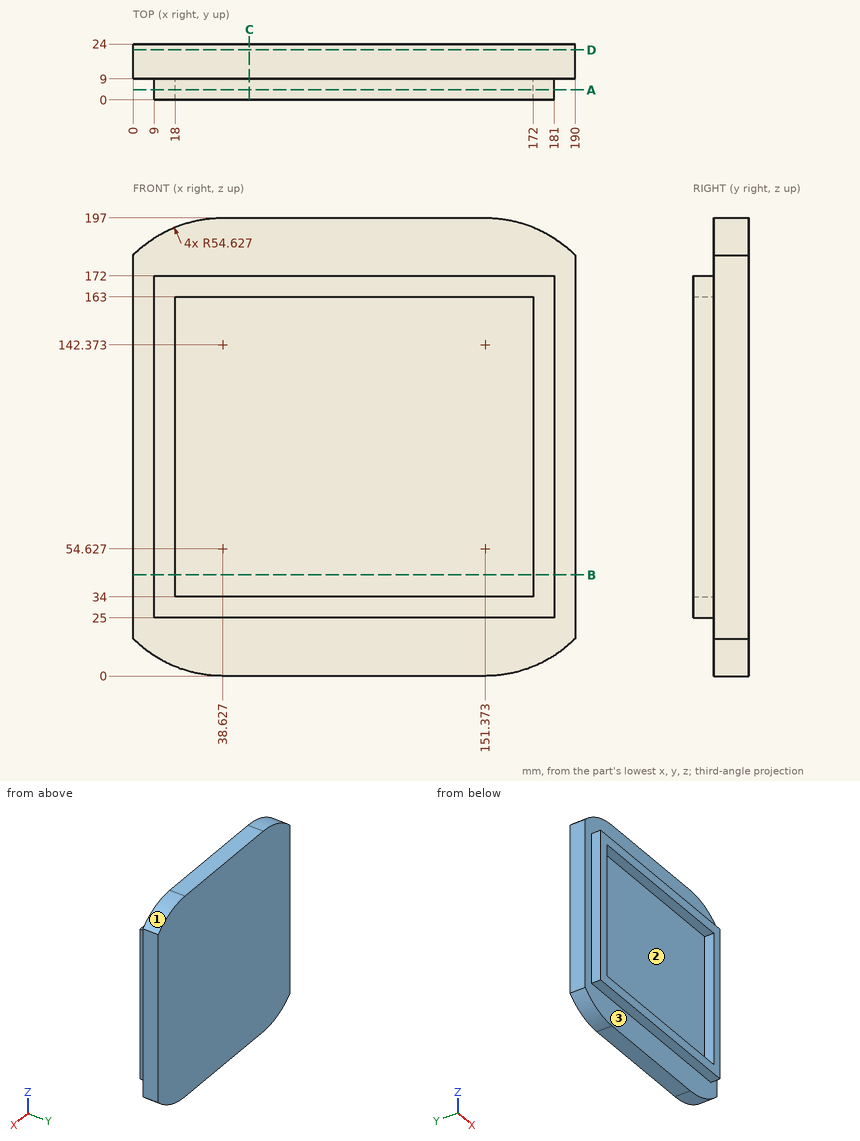
Source: three-view drawing plus pictorial views. Frame: mm from the lowest corner of the part. Round coordinates to 2 decimals unless told otherwise and drop trailing zeros. Write each loop counter-clockwise with the first axis right and the second up, starting at its lowest first coordinate (ties: lowest second). Pieces come first, ordered by that corner, then holes. Notation, with made-up numbers: M 54,67.25 L 100,67.25 A15 ccw 100,96.25 Z; hole C 51.5,-6 d3. An arc over 180 degrees is marked long. Use CSV: the item, a comma, the result in double quotes. Start each with the question number.
Q1. Line query: line 1 (X direction, y = 7.75, z = 73.5); line 2 (Z direction, x = 131, y = 4); line 3 (Y direction, x = 159, z = 137.5). Output: solid intervals per line, ascending. Write a range as from..to.
Q2. First-contact query: P1, Ø12, axis at x = 122.5, y = 14.5, coming from the -Z side; P2, Ø4.5, axis at x = 57, y = 3, coming from the -Z side; P3, Ø4.5, axis at x = 102.5, y = 5.5, coming from the +Z side; P4, Ø7, axis at y = 4.5, z = 91.5, coming from the +X side. Flat tips, straight axial feed; report the tip coordinate or a pass-through.
Q3. Pull-direction query (Z, two-part tool) for the marked faces 1, 2 and 3; classes: +Z half, -Z half, draft (parallel to the pull), parting line (faces both ways), or undercut.
Q4. Cut plane A-A on y = 4.25. Output: boundary loops of the cut face in (x, z).
Q5. Cut plane D-D on y = 21.5. Output: boundary loops of the cut face in (x, z) (1 decimal), plus the area to 3 significant figures.
Q6. Cut plane C-C on x = 50. Output: boundary loops of the cut face in (y, z), plus the area to 3 significant figures.
Q7. Cut plane B-B on z = 43.5. Output: boundary loops of the cut face in (x, y), plus the area to 3 significant figures.
Results found:
1,line 1,"9..18, 172..181"
1,line 2,"25..34, 163..172"
1,line 3,"9..24"
2,P1,"z = 0"
2,P2,"z = 25"
2,P3,"z = 172"
2,P4,"x = 181"
3,face 1,"+Z half"
3,face 2,"undercut"
3,face 3,"draft"
4,outline,"M 9,25 L 181,25 L 181,172 L 9,172 Z; hole M 18,34 L 172,34 L 172,163 L 18,163 Z"
5,outline,"M 0,16 A54.6 ccw 38.6,0 L 151.4,0 A54.6 ccw 190,16 L 190,181 A54.6 ccw 151.4,197 L 38.6,197 A54.6 ccw 0,181 Z"
5,area,"36,700 mm^2"
6,outline,"M 0,25 L 9,25 L 9,0 L 24,0 L 24,197 L 9,197 L 9,172 L 0,172 L 0,163 L 9,163 L 9,34 L 0,34 Z"
6,area,"3,120 mm^2"
7,outline,"M 0,9 L 9,9 L 9,0 L 18,0 L 18,9 L 172,9 L 172,0 L 181,0 L 181,9 L 190,9 L 190,24 L 0,24 Z"
7,area,"3,010 mm^2"
